Autodesk Inventor part; units mm, degrees
ref_plane "YZ Plane" through (0, 0, 0) normal (1, 0, 0) x (0, 1, 0)
ref_plane "XZ Plane" through (0, 0, 0) normal (0, 1, 0) x (-1, 0, 0)
ref_plane "XY Plane" through (0, 0, 0) normal (0, 0, 1) x (1, 0, 0)
sketch "cover" plane through (0, 0, 0) normal (0, 0, 1) x (1, 0, 0)
  line L0 (20.7283, -19.2532) -> (20.7283, 19.7468)
  line L1 (20.7283, 19.7468) -> (-21.2598, 19.7468)
  line L2 (-21.2598, 19.7468) -> (-21.2598, -20.2532)
  line L3 (-21.2598, -20.2532) -> (20.7283, 19.7468) construction
  line L4 (20.7283, -19.2532) -> (-21.2598, 19.7468) construction
  line L5 (21.7283, -19.2532) -> (21.7283, 20.7468)
  line L6 (21.7283, 20.7468) -> (-22.2598, 20.7468)
  line L7 (-22.2598, 20.7468) -> (-22.2598, 19.7468)
  line L8 (-22.2598, 19.7468) -> (-22.2598, -20.2532)
  line L9 (-21.2598, -20.2532) -> (-22.2598, -20.2532)
  line L10 (20.7283, -19.2532) -> (21.7283, -19.2532)
  point P0 (0, 0)
  dimension "d56" = 42
  dimension "d57" = 40
  dimension "d92" = 1
  dimension "d95" = 1
  dimension "d100" = 1
extrude "Extrusion8" add sketch "cover" along normal blind 44.4
fillet "Fillet5" radius 2 1 edges at (-21.2598, 19.7468, 22.2)
fillet "Fillet6" radius 2 1 edges at (20.7283, 19.7468, 22.2)
fillet "Fillet7" radius 2 1 edges at (-22.2598, 20.7468, 22.2)
fillet "Fillet8" radius 2 1 edges at (21.7283, 20.7468, 22.2)
equation "\"d56\" = wallw"
equation "\"d57\" = wallh - base_slots_depth"
equation "\"d92\" = 0.5 * baseextra"
equation "\"d95\" = d92"
equation "\"d100\" = d92"
equation "\"d93\" = wall1_thick + gap1 + wall2_thick"
equation "\"d96\" = cornerrad"
equation "\"d97\" = cornerrad"
equation "\"d98\" = cornerrad"
equation "\"d99\" = cornerrad"
equation "\"printer3dtolerance\" = 0.12"
equation "\"wallw\" = 42"
equation "\"wallh\" = 44"
equation "\"cornerrad\" = 2"
equation "\"baseextra\" = 2"
equation "\"wall1_thick\" = 8"
equation "\"wall2_thick\" = 6.4"
equation "\"wall3_thick\" = 4"
equation "\"wall1slot\" = 8.12"
equation "\"wall2slot\" = 6.52"
equation "\"wall3slot\" = 4.12"
equation "\"gap1\" = 30"
equation "\"gap2\" = 28"
equation "\"baseh\" = 79.12"
equation "\"basew\" = 44"
equation "\"base_thick\" = 6"
equation "\"base_slots_depth\" = 4"
equation "\"d26\" = 8.12"
equation "\"d27\" = 42"
equation "\"d28\" = 44"
equation "\"d29\" = 28"
equation "\"d31\" = 4.12"
equation "\"d32\" = 6.52"
equation "\"d33\" = 79.12"
equation "\"d39\" = 8.12"
equation "\"d40\" = 42"
equation "\"d41\" = 44"
equation "\"d48\" = 8.12"
equation "\"d49\" = 42"
equation "\"d50\" = 8.12"
equation "\"d51\" = 42"
equation "\"d52\" = 44"
equation "\"d53\" = 44"
equation "\"d71\" = 8.12"
equation "\"d72\" = 42"
equation "\"d73\" = 2"
equation "\"d74\" = 44"
equation "\"distancefrombottom\" = 34"
equation "\"servosmallcircledia\" = 5.92"
equation "\"servo9gw\" = 22.8"
equation "\"servomountsquare\" = 6"
equation "\"servopolygonl\" = 5.92"
equation "\"servopolygonr\" = 6.12"
equation "\"distancefromleft\" = 26"
equation "\"servobigcircledia\" = 11.62"
equation "\"servomounth\" = 4"
equation "\"wall3slotd\" = 2"
equation "\"wall3slotw\" = 36"
equation "\"adapterh\" = 16"
equation "\"adapterw\" = 32"
equation "\"wall3slotd_1\" = 2"
properties part number "back-cover" material "Wood (Oak)"
Can you work these out from the model? Positions are in its coordinate system, mm. A direction names the side the tool comes from. Coordinates: 2 decimals unless noted, no trailing zeros. Order: outer loops, then holes, each group sorted by start corner. A loop starts at its lowest first (then second) coordinate and runs counter-clockwise, first axis right, second up. Notation, with made-up numbers: (62, 76.25) - (100, 76.25) arc R30 cw to (100, 98.25) - close; hole circle Ø4 at (45, -38). An arc over 180 degrees is marked (long way). Answer in a Markdown table with one row per item.
1. If I drill on line 1 along X through (y, z) = (-12, 14); line 2 along Y through (x, z) = (6.5, 14); line 3 along Y through (x, z) = (19.5, 7), over which ranges is the centre line in solid material (lowest first)?
Reply:
| item | result |
|---|---|
| line 1 | x = -22.26 to -21.26, 20.73 to 21.73 |
| line 2 | y = 19.75 to 20.75 |
| line 3 | y = 19.59 to 20.75 |
2. For faces 5 (the flat face through (20.728, -1, 22)), 6 (the flat face through (-22.26, 0, 22)), which set-ups out of +Z, -Z, +X, -X, +Y, -Y let a thin tool reach every point of the face, with its end or its side?
Reply:
| item | result |
|---|---|
| face 5 | +Z, -Z, -Y |
| face 6 | +Z, -Z, -X, +Y, -Y |
3. If we mould it in two halves opening along X, with no side actions, what happens to faces 1 (the flat face through (0, 20.747, 22)), 2 (the flat face through (21.728, -1, 22)), 3 (the cylindrical face through (20.2, 19.1, 22.5)), 4 (the cylindrical face through (-20.658, 19.176, 22.511))? For each: pulls with the +X half, pulls with the -X half, needs draft (parallel to the pull), parting line crosses it, or undercut.
Reply:
| item | result |
|---|---|
| face 1 | needs draft |
| face 2 | pulls with the +X half |
| face 3 | undercut |
| face 4 | undercut |
4. For pin 1 (1.1 mm diameter, centred on x = 21.5, z = 29.5, fed in from -Y); pin 2 (11.5 mm diameter, centred on x = -7.5, z = 30, fed in from -Y), each with a flat end and sliding along its axis, tell me the tip position at first contact or that it passes through.
Reply:
| item | result |
|---|---|
| pin 1 | stops at y = -19.25 |
| pin 2 | stops at y = 19.75 |
5. Suppose I cut it at A-A (y = 15). Please give me the cut outline in (x, z), and give its area (3 significant figures).
Reply:
| item | result |
|---|---|
| outline | (-22.26, 0) - (-21.26, 0) - (-21.26, 44.4) - (-22.26, 44.4) - close; (20.73, 0) - (21.73, 0) - (21.73, 44.4) - (20.73, 44.4) - close |
| area | 88.8 mm^2 |
6. Suppose I cut it at B-B (x = -13.5). Please give me the cut outline in (y, z).
Reply:
| item | result |
|---|---|
| outline | (19.75, 0) - (20.75, 0) - (20.75, 44.4) - (19.75, 44.4) - close |
